```python
from build123d import *

# Parameters (mm, degrees)
BOSS_EXTRUDE3_DEPTH = 7.62
SKETCH6_W           = 108.110429846
SKETCH6_H           = 40.078189215
SKETCH6_W_2         = 39.947123602
SKETCH6_H_2         = 20.1313586
CUT_EXTRUDE5_DEPTH  = 7.62


with BuildPart() as part:
    # Sketch2 → Boss-Extrude3 (new body)
    with BuildSketch(Plane.XY):
        with BuildLine():
            Line((96.126803593, -12.916705994), (94.17394782, -10.963850221))
            add(Edge.make_bspline(
                [(75.252666665, 12.699131487), (83.268217656, -0.404579698), (94.17394782, -10.963850221)],
                knots=[0, 0, 0, 1, 1, 1], degree=2))
            ThreePointArc((75.252666665, 12.699131487), (-45.402140278, 61.342297308), (-34.129845534, -68.259691067))
            Line((-34.129845534, -68.259691067), (-34.129845534, -119.480702222))
            Line((-34.129845534, -119.480702222), (45.224618014, -119.480702222))
            Line((45.224618014, -119.480702222), (45.224618014, -84.189817543))
            Line((45.224618014, -84.189817543), (7.693042244, -68.259691067))
            Line((7.693042244, -68.259691067), (7.693042244, -31.273550257))
            Line((7.693042244, -31.273550257), (76.316654675, -31.273550257))
            Line((76.316654675, -31.273550257), (76.316654675, -21.354495246))
            Line((76.316654675, -21.354495246), (93.197519934, -21.354495246))
            ThreePointArc((93.197519934, -21.354495246), (97.451679759, -18.688706069), (96.907945902, -13.697848303))
            Line((96.907945902, -13.697848303), (96.126803593, -12.916705994))
        make_face()
    extrude(amount=BOSS_EXTRUDE3_DEPTH)

    # Sketch6 → Cut-Extrude5 (cut)
    with BuildSketch(Plane.XY.offset(7.62)):
        with Locations((-0.597955264, 25.976582243)):
            Rectangle(SKETCH6_W, SKETCH6_H)
        with Locations((8.508452954, -10.0656793)):
            Rectangle(SKETCH6_W_2, SKETCH6_H_2)
    extrude(amount=-CUT_EXTRUDE5_DEPTH, mode=Mode.SUBTRACT)


solid = part.part
```
Here's how the part is built. I have some questions about the finished solid (model axes, mm). A direction names the side the tool comes from. Give positions to 0.01 mm unless a question says otherwise; leave off trailing zeros. Loops run counter-clockwise (first coordinate to the right, second up) from the corner with the lowest first, then second, coordinate; pieces in that order, holes last. Notation, with made-up numbers: (0.5, -10) -> (18.5, -10) arc R13 ccw to (18.5, 9) -> close; hole circle Ø4 at (89, 69.25). An arc over 180 degrees is marked (long way). Use one line per item in the form item = value. Start each with the question number.
1) Imagine slicing it at D-D (y = -17.5). Please give me the cut outline in (x, z).
2) Imagine slicing it at B-B (x = 26). Please give me the cut outline in (y, z).
3) Thinking about a two-plate mould opening in Y: for faces 1 (the face through (-43.631, 62.614, 3.757)), 2 (the face through (-34.13, -94, 4)), 3 (the face through (28.482, -10, 4)), which applies, +Y half, -Y half, draft (parallel to the pull), parting line (faces both ways), or undercut?
4) Imagine slicing it at C-C (x = -36.5). Please give me the cut outline in (y, z), then the cut area to 3 significant figures.
5) Imagine slicing it at A-A (x = 0). Please give me the cut outline in (y, z).
6) For P1, Ø4, axis at x = 12, z = 2.5, coming from the +Y side; P2, Ø2.5, axis at y = 25, z = 3, coming from the -X side; P3, Ø4, axis at y = -58, z = 4, coming from the +X side; P4, Ø1.5, axis at x = -29.5, y = 55, coming from the -Z side, each with a flat end and sliding along its axis, tell me the tip position at first contact or that it passes through.
7) Which directions (+Z, -Z, +X, -X, +Y, -Y) give clear straight access to the entire face, cutting with the end or side of a thin tool? Please do faces 4 (the face through (5, -119.481, 4)), 5 (the face through (85, -21.354, 4)), 6 (the face through (7.693, -50, 4)), 7 (the face through (-7, -42, 7.62)), 8 (the face through (8, 0, 4)).
8) Please list where these lines run through material, in increasing order: line 1 along X through (y, z) = (-95, 0.75); line 2 along Y through (x, z) = (-4, 0.75); line 3 along X through (y, z) = (-15, 6.25).
Check values:
q1.outline = (-74.28, 0) -> (-11.47, 0) -> (-11.47, 7.62) -> (-74.28, 7.62) -> close; (28.48, 0) -> (97.84, 0) -> (97.84, 7.62) -> (28.48, 7.62) -> close
q2.outline = (-119.48, 0) -> (-76.03, 0) -> (-76.03, 7.62) -> (-119.48, 7.62) -> close; (-31.27, 0) -> (-20.13, 0) -> (-20.13, 7.62) -> (-31.27, 7.62) -> close; (0, 0) -> (5.94, 0) -> (5.94, 7.62) -> (0, 7.62) -> close; (46.02, 0) -> (71.75, 0) -> (71.75, 7.62) -> (46.02, 7.62) -> close
q3.face_1 = parting line
q3.face_2 = draft
q3.face_3 = undercut
q4.outline = (-67.02, 0) -> (5.94, 0) -> (5.94, 7.62) -> (-67.02, 7.62) -> close; (46.02, 0) -> (67.02, 0) -> (67.02, 7.62) -> (46.02, 7.62) -> close
q4.area = 716 mm^2
q5.outline = (-119.48, 0) -> (-20.13, 0) -> (-20.13, 7.62) -> (-119.48, 7.62) -> close; (0, 0) -> (5.94, 0) -> (5.94, 7.62) -> (0, 7.62) -> close; (46.02, 0) -> (76.32, 0) -> (76.32, 7.62) -> (46.02, 7.62) -> close
q6.P1 = 75.66
q6.P2 = -72.53
q6.P3 = 7.69
q6.P4 = 0
q7.face_4 = +Z, -Z, +X, -X, -Y
q7.face_5 = +Z, -Z, +X, -Y
q7.face_6 = +Z, -Z, +X
q7.face_7 = +Z, +X, -X, +Y, -Y
q7.face_8 = +Z, -Z
q8.line_1 = -34.13 to 45.22
q8.line_2 = -119.48 to -20.13, 0 to 5.94, 46.02 to 76.21
q8.line_3 = -74.83 to -11.47, 28.48 to 97.64
